Model file for the job. Use its own axes, mm. Coordinates: 2 decimals unless noted, no trailing zeros. Write each loop counter-clockwise with the first axis right and the second up, starting at its lowest first coordinate (ties: lowest second). Pieces come first, ordered by that corner, then holes. Notation, with made-up numbers: M -8,7 L 29,7 A34 ccw 29,42 Z; hole C 28.25,66 d8. An arc over 180 degrees is marked long. Put each result on its own line as item: value. Start each with the question number.
Q1. Cut at B-B (x = 6.6). Write the cut outline in (y, z), then the cut area to 3 significant figures.
Q2. Drill centre lines: line 1 along Z through (x, y) = (-0.55, -6.6); line 2 along Z through (x, y) = (6.6, 0.2); line 3 along Z through (x, y) = (7.25, 0.5). Where is each one in solid material? Low to high.
Q3. Cut at A-A (z = 125). Write the cut outline in (x, y).
Q4. Drop flat-ended pins along their axis: pin 1 (1.5 mm diameter, centred on x = 5.5, z = 128.5, fed in from -Y); pin 2 (7.5 mm diameter, centred on y = -6.6, z = 62.5, fed in from +X); pin 3 (6 mm diameter, centred on x = 2.5, z = 141, fed in from +Y) (3 decimals); pin 4 (4 mm diameter, centred on y = -6.6, z = 187.5, fed in from +X). Give the stop position or say it passes through.
Q5. Cut at C-C (y = -6.6). Write the cut outline in (x, z).
Q6. Cut at D-D (z = 187.5). Write the cut outline in (x, y), then the cut area to 3 significant figures.
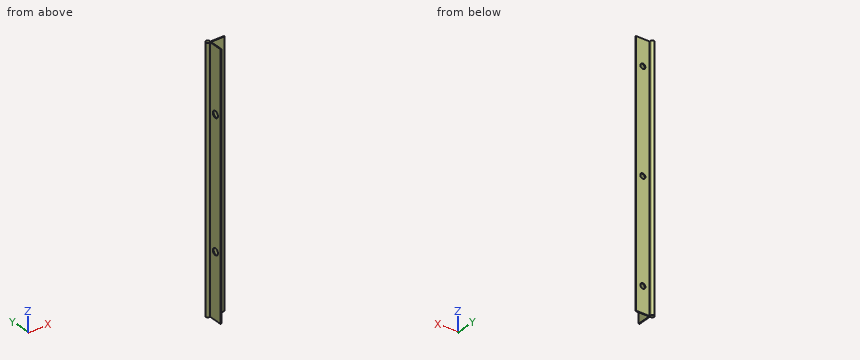
```python
from build123d import *

# Parameters (mm, degrees)
F1_DEPTH = 250
F2_R     = 2.5
F3_DEPTH = 14.001
F4_R     = 3.25
F5_DEPTH = 3.601


with BuildPart() as f1:
    # F0 (on Top) → F1 (new body)
    with BuildSketch(Plane.XY):
        with BuildLine():
            ThreePointArc((0, 1.8), (-3.072792, 3.072792), (-1.8, 0))
            ThreePointArc((-1.8, 0), (-0.527208, 0.527208), (0, 1.8))
        make_face()
        with BuildLine():
            Line((0, -13.2), (0, 0))
            Line((0, 0), (13.2, 0))
            Line((13.2, 0), (13.2, 0.8))
            Line((13.2, 0.8), (0, 0.8))
            Line((0, 0.8), (0, 1.8))
            ThreePointArc((0, 1.8), (-0.527208, 0.527208), (-1.8, 0))
            Line((-1.8, 0), (-0.8, 0))
            Line((-0.8, 0), (-0.8, -13.2))
            Line((-0.8, -13.2), (0, -13.2))
        make_face()
    extrude(amount=F1_DEPTH)

    # F2 (on face) → F3 (cut, through all)
    with BuildSketch(Plane(origin=(0, 0.8, 0), x_dir=(-1, 0, 0), z_dir=(0, 1, 0))):
        with Locations((-6.6, 25)):
            Circle(F2_R)
        with Locations((-6.6, 125)):
            Circle(F2_R)
        with Locations((-6.6, 225)):
            Circle(F2_R)
    extrude(amount=-F3_DEPTH, mode=Mode.SUBTRACT)

    # F4 (on face) → F5 (cut, through all)
    with BuildSketch(Plane.YZ):
        with Locations((-6.6, 187.5)):
            Circle(F4_R)
        with Locations((-6.6, 62.5)):
            Circle(F4_R)
    extrude(amount=-F5_DEPTH, mode=Mode.SUBTRACT)


solid = f1.part
```
Computed values:
1. outline: M 0,0 L 0.8,0 L 0.8,22.5 L 0,22.5 Z; M 0,27.5 L 0.8,27.5 L 0.8,122.5 L 0,122.5 Z; M 0,127.5 L 0.8,127.5 L 0.8,222.5 L 0,222.5 Z; M 0,227.5 L 0.8,227.5 L 0.8,250 L 0,250 Z
1. area: 188 mm2
2. line 1: 0 to 59.25, 65.75 to 184.25, 190.75 to 250
2. line 2: 0 to 22.5, 27.5 to 122.5, 127.5 to 222.5, 227.5 to 250
2. line 3: 0 to 22.59, 27.41 to 122.59, 127.41 to 222.59, 227.41 to 250
3. outline: M -1.8,0 L -0.8,0 L -0.8,-13.2 L 0,-13.2 L 0,0 L 4.1,0 L 4.1,0.8 L 0,0.8 L 0,1.8 A1.8 ccw long Z; M 9.1,0 L 13.2,0 L 13.2,0.8 L 9.1,0.8 Z
4. pin 1: y = 0
4. pin 2: x = 0
4. pin 3: y = 3.045
4. pin 4: through
5. outline: M -0.8,0 L 0,0 L 0,59.25 L -0.8,59.25 Z; M -0.8,65.75 L 0,65.75 L 0,184.25 L -0.8,184.25 Z; M -0.8,190.75 L 0,190.75 L 0,250 L -0.8,250 Z
6. outline: M -1.8,0 L -0.8,0 L -0.8,-3.35 L 0,-3.35 L 0,0 L 13.2,0 L 13.2,0.8 L 0,0.8 L 0,1.8 A1.8 ccw long Z; M -0.8,-13.2 L 0,-13.2 L 0,-9.85 L -0.8,-9.85 Z
6. area: 26.8 mm2
